from build123d import *

# Parameters (mm, degrees)
SKETCH1_W           = 170
SKETCH1_H           = 120
SKETCH1_W_2         = 40
SKETCH1_H_2         = 12.7
SKETCH1_W_3         = 60
SKETCH1_H_3         = 40
BOSS_EXTRUDE1_DEPTH = 12.7
SKETCH2_R           = 4
SKETCH2_W           = 12.7
SKETCH2_H           = 40
CUT_EXTRUDE1_DEPTH  = 12.7


with BuildPart() as part:
    # Sketch1 → Boss-Extrude1 (new body)
    with BuildSketch(Plane(origin=(0, 0, 0), x_dir=(0, 0, -1), z_dir=(1, 0, 0))):
        Rectangle(SKETCH1_W, SKETCH1_H)
        with Locations((-15, -66.35)):
            Rectangle(SKETCH1_W_2, SKETCH1_H_2)
        with Locations((-115, 0)):
            Rectangle(SKETCH1_W_3, SKETCH1_H_3)
    extrude(amount=BOSS_EXTRUDE1_DEPTH)

    # Sketch2 → Cut-Extrude1 (cut)
    with BuildSketch(Plane(origin=(12.7, 0, 0), x_dir=(0, 0, -1), z_dir=(1, 0, 0))):
        with Locations((-115, 0)):
            Circle(SKETCH2_R)
        with Locations((-78.65, -40)):
            Rectangle(SKETCH2_W, SKETCH2_H)
        with Locations((78.65, -40)):
            Rectangle(SKETCH2_W, SKETCH2_H)
    extrude(amount=-CUT_EXTRUDE1_DEPTH, mode=Mode.SUBTRACT)


solid = part.part
The listing builds one solid part. Answer for the finished solid, in the listing's coordinates (mm). A direction names the side the tool comes from. Coordinates: 2 decimals unless noted, no trailing zeros. Write each loop counter-clockwise with the first axis right and the second up, starting at its lowest first coordinate (ties: lowest second). Pieces come first, ordered by that corner, then holes. Notation, with made-up numbers: (29.5, 30) - (47.5, 30) arc R23 ccw to (47.5, 65) - close; hole circle Ø5 at (81, -22.75). An arc over 180 degrees is marked (long way). Put each result on its own line as item: value.
1. The part is cut by section D-D on z = 64.5. Give the vertices of the cut face in (x, y).
Answer sheet:
outline: (0, -60) - (12.7, -60) - (12.7, 60) - (0, 60) - close
2. Find the intervals of material crossed by line 1 along Y through (x, z) = (7.5, 115); line 2 along Y through (x, z) = (10.75, 104); line 3 along Y through (x, z) = (2.5, 116), in increasing order. Write a range as from..to.
Answer sheet:
line 1: y = -20..-4, 4..20
line 2: y = -20..20
line 3: y = -20..-3.87, 3.87..20
3. Determine the mould class of faces 6 (the face through (6, -40, -72.3)), 7 (the face through (6.439, -1.532, 111.305)), 8 (the face through (6, -60, 54)) for opening direction Z: pulls with the +Z half, pulls with the -Z half, needs draft (parallel to the pull), parting line crosses it, or undercut.
Answer sheet:
face 6: pulls with the -Z half
face 7: undercut
face 8: needs draft
4. The part is cut by section B-B on z = 115. Give the vertices of the cut face in (x, y).
Answer sheet:
outline: (0, -20) - (12.7, -20) - (12.7, -4) - (0, -4) - close; (0, 4) - (12.7, 4) - (12.7, 20) - (0, 20) - close
5. The part is cut by section A-A on y = 0. Give the vertices of the cut face in (x, z).
Answer sheet:
outline: (0, -85) - (12.7, -85) - (12.7, 111) - (0, 111) - close; (0, 119) - (12.7, 119) - (12.7, 145) - (0, 145) - close
6. A tool of negligible diameter and unlimited length cuts with its end or side. For faces 1 (the face through (6, -72.7, 15)), 2 (the face through (6, -20, -79)), 3 (the face through (0, -5, 6)), 4 (the face through (6, -40, 72.3)), 5 (the face through (6, 40, 85)), from which of +Z, -Z, +X, -X, +Y, -Y can it reach the whole face along a straight path? Write none if from no direction.
Answer sheet:
face 1: +Z, -Z, +X, -X, -Y
face 2: -Z, +X, -X, -Y
face 3: +Z, -Z, -X, +Y, -Y
face 4: +Z, +X, -X, -Y
face 5: +Z, +X, -X, +Y
7. Flat-ended cylindrical pins translate along their axes: pin 1 Ø4 at (x, y) = (9.5, -69) entering from +Z; pin 2 Ø5 at (x, z) = (6.5, 45) entering from -Y; pin 3 Ø3 at (x, y) = (6.5, 33) entering from +Z; pin 4 Ø5 at (y, z) = (0, 115) entering from -X. Find the tip coordinate at first contact, or state that the pin passes through.
Answer sheet:
pin 1: stops at z = 35
pin 2: stops at y = -60
pin 3: stops at z = 85
pin 4: passes through
8. The part is cut by section C-C on x = 5.5. Give the vertices of the cut face in (y, z).
Answer sheet:
outline: (-72.7, -5) - (-60, -5) - (-60, -72.3) - (-20, -72.3) - (-20, -85) - (60, -85) - (60, 85) - (20, 85) - (20, 145) - (-20, 145) - (-20, 72.3) - (-60, 72.3) - (-60, 35) - (-72.7, 35) - close; hole circle Ø8 at (0, 115)
